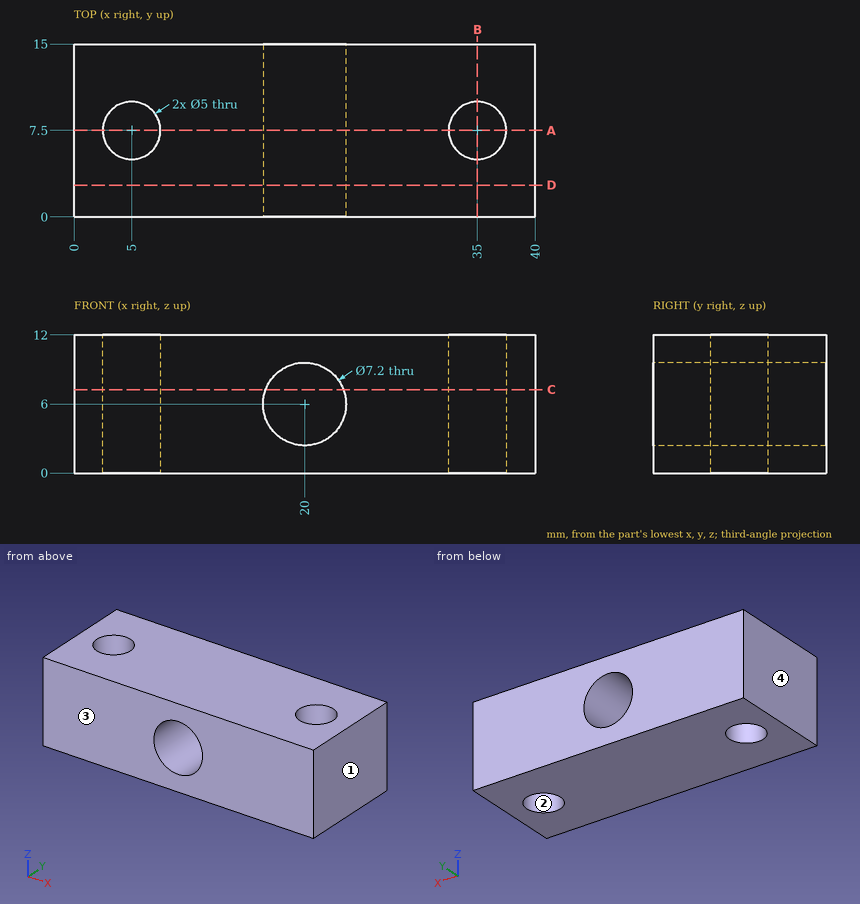
The figure shows three views and two pictorial views of one solid part (mm, origin at its lowest corner). Answer the questions. Give positions to 0.01 mm unless a question says otherwise; leave off trailing zeros. Write each loop counter-clockwise with the first axis right and the second up, starting at its lowest first coordinate (ties: lowest second). Pieces come first, ordered by that corner, then holes. Notation, with made-up numbers: (59.5, 47.25) - (110.5, 47.25) arc R25 cw to (110.5, 75.25) - close; hole circle Ø9 at (73, 44). An arc over 180 degrees is marked (long way). Use one line per item in the form item = value. Start each with the question number.
1) Consider line 1 along X through (y, z) = (3.75, 6); line 2 along Y through (x, z) = (5, 3.25); line 3 along Z through (x, y) = (20, 7.75). Determine where each line is inside the solid, lowest interval first. Write a range as from..to.
2) Find section A-A on y = 7.5. Determine the outline of the cut face in (x, z), plus the area to 3 significant figures.
3) Find section B-B on x = 35. Determine the outline of the cut face in (y, z).
4) The mould has two halves that part along X. Classify the marked faces 1, 2, 3 and 4: pulls with the +X half, pulls with the -X half, needs draft (parallel to the pull), parting line crosses it, or undercut.
5) Find section C-C on z = 7.25. Determine the outline of the cut face in (x, y), plus the area to 3 significant figures.
6) Find section D-D on y = 2.75. Determine the outline of the cut face in (x, z).
Geometry results:
q1.line_1 = 0..16.4, 23.6..40
q1.line_2 = 0..5, 10..15
q1.line_3 = 0..2.4, 9.6..12
q2.outline = (0, 0) - (2.5, 0) - (2.5, 12) - (0, 12) - close; (7.5, 0) - (32.5, 0) - (32.5, 12) - (7.5, 12) - close; (37.5, 0) - (40, 0) - (40, 12) - (37.5, 12) - close; hole circle Ø7.2 at (20, 6)
q2.area = 319 mm2
q3.outline = (0, 0) - (5, 0) - (5, 12) - (0, 12) - close; (10, 0) - (15, 0) - (15, 12) - (10, 12) - close
q4.face_1 = pulls with the +X half
q4.face_2 = undercut
q4.face_3 = needs draft
q4.face_4 = pulls with the -X half
q5.outline = (0, 0) - (16.62, 0) - (16.62, 15) - (0, 15) - close; (23.38, 0) - (40, 0) - (40, 15) - (23.38, 15) - close; hole circle Ø5 at (5, 7.5); hole circle Ø5 at (35, 7.5)
q5.area = 459 mm2
q6.outline = (0, 0) - (40, 0) - (40, 12) - (0, 12) - close; hole circle Ø7.2 at (20, 6)
